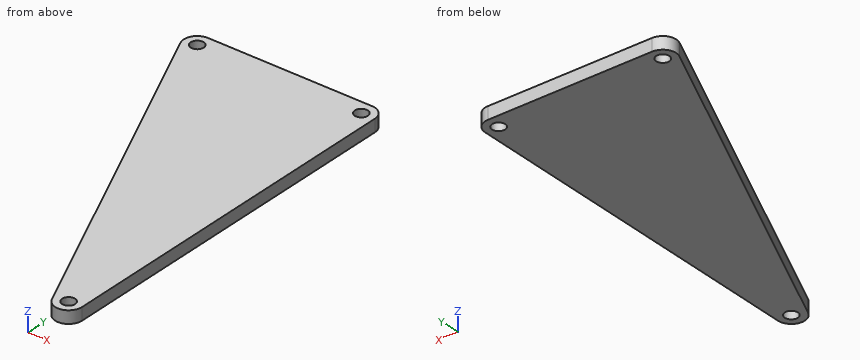
```python
from build123d import *

# Parameters (mm, degrees)
SKETCH1_R           = 4.32
SKETCH1_R_2         = 2.1
BOSS_EXTRUDE1_DEPTH = 4


with BuildPart() as part:
    # Sketch1 → Boss-Extrude1 (new body)
    with BuildSketch(Plane.XY):
        with BuildLine():
            Line((52.7, 4.32), (0, 4.32))
            ThreePointArc((0, 4.32), (3.054701295, 3.054701295), (4.32, 0))
            ThreePointArc((4.32, 0), (0.907798653, -4.223541358), (-3.938472965, -1.775057943))
            Line((-3.938472965, -1.775057943), (48.761527035, -118.705057943))
            ThreePointArc((48.761527035, -118.705057943), (51.792201347, -112.706458642), (57.02, -116.93))
            Line((57.02, -116.93), (57.02, 0))
            ThreePointArc((57.02, 0), (49.645298705, -3.054701295), (52.7, 4.32))
        make_face()
        Circle(SKETCH1_R)
        Circle(SKETCH1_R_2, mode=Mode.SUBTRACT)
        with Locations((52.7, 0)):
            Circle(SKETCH1_R)
        with Locations((52.7, 0)):
            Circle(SKETCH1_R_2, mode=Mode.SUBTRACT)
        with Locations((52.7, -116.93)):
            Circle(SKETCH1_R)
        with Locations((52.7, -116.93)):
            Circle(SKETCH1_R_2, mode=Mode.SUBTRACT)
    extrude(amount=BOSS_EXTRUDE1_DEPTH)


solid = part.part
```
The model under review builds one solid part; all positions refer to its coordinate system, in mm. Round coordinates to 2 decimals unless told otherwise and drop trailing zeros. Order: outer loops, then holes, each group sorted by start corner. A loop starts at its lowest first (then second) coordinate and runs counter-clockwise, first axis right, second up. Notation, with made-up numbers: (-38.5, 2) - (-14.5, 2) arc R12 ccw to (-14.5, 14) - close; hole circle Ø10 at (37, 73.5). An arc over 180 degrees is marked (long way). Answer in a Markdown table with one row per item.
(1) For line 1 (Y direction, x = 52.7, z = 1.15); line 2 (Y direction, x = 0, z = 0.9); line 3 (Y direction, x = 7, z = 2.95), list the stretches that pass through material, from the lowest coordinate up. Write a range as from..to.
Result set:
| item | result |
|---|---|
| line 1 | y = -121.25..-119.03, -114.83..-2.1, 2.1..4.32 |
| line 2 | y = -10.51..-2.1, 2.1..4.32 |
| line 3 | y = -26.05..4.32 |
(2) Take a section at A-A on z = 1.5. Write out the cut boundary in (x, y).
Result set:
| item | result |
|---|---|
| outline | (-3.94, -1.78) - (48.76, -118.71) arc R4.32 ccw to (57.02, -116.93) - (57.02, 0) arc R4.32 ccw to (52.7, 4.32) - (0, 4.32) arc R4.32 ccw to start; hole circle Ø4.2 at (0, 0); hole circle Ø4.2 at (52.7, -116.93); hole circle Ø4.2 at (52.7, 0) |
(3) Take a section at C-C on y = -27. Write out the cut boundary in (x, z).
Result set:
| item | result |
|---|---|
| outline | (7.43, 0) - (57.02, 0) - (57.02, 4) - (7.43, 4) - close |
(4) Take a section at B-B on x = 9.5. Write out the cut boundary in (y, z).
Result set:
| item | result |
|---|---|
| outline | (-31.59, 0) - (4.32, 0) - (4.32, 4) - (-31.59, 4) - close |
(5) Clearance check with a flat-ended pin moving along its axis: P1, Ø2, axis at x = 23, y = -15, coming from the -Z side. State where the tip first meets the part, or that it passes through.
Result set:
| item | result |
|---|---|
| P1 | stops at z = 0 |
